Source: three-view drawing plus pictorial views. Frame: mm from the lowest corner of the part. Coordinates: 2 decimals unless noted, no trailing zeros. Order: outer loops, then holes, each group sorted by start corner. A loop starts at its lowest first (then second) coordinate and runs counter-clockwise, first axis right, second up. Notation, with made-up numbers: (26.5, 61) -> (85.5, 61) arc R25 ccw to (85.5, 93) -> close; hole circle Ø5 at (-22.5, 69.5). An arc over 180 degrees is marked (long way). Use one line per item in the form item = value. Start each with the question number.
1) Section query B-B on y = 55. Output: boundary loops of the cut face in (x, z), then the cut area to 3 significant figures.
2) Pin query (flat end, axial travel): pin 1 (2 mm diameter, centred on y = 11.2, z = 2.5, fed in from -X). Return the tip coordinate at first contact, or that it passes through.
3) Ray query, line 1 along X through (y, z) = (26.5, 2.3); line 2 along X through (y, z) = (52, 3.3); line 3 along Y through (x, z) = (41.3, 2.5). Return the intervals inside material, ascending.
4) Section query A-A on x = 36.5. Output: boundary loops of the cut face in (y, z).
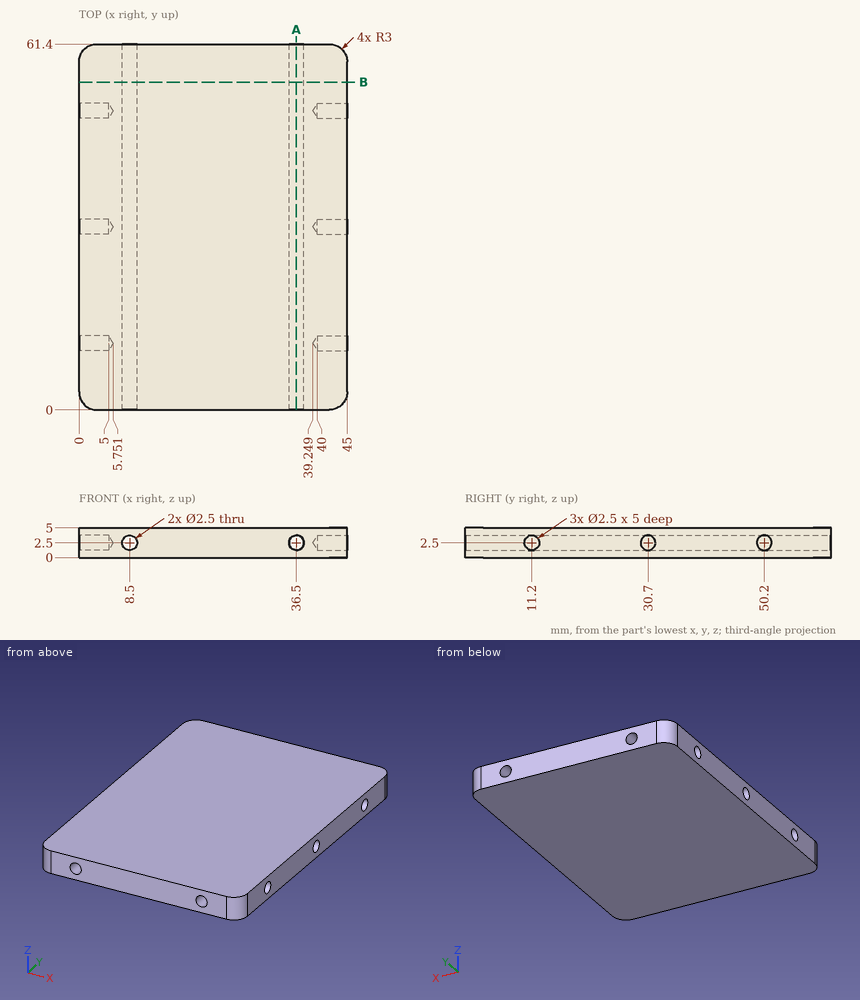
Answers below:
q1.outline = (0, 0) -> (45, 0) -> (45, 5) -> (0, 5) -> close; hole circle Ø2.5 at (8.5, 2.5); hole circle Ø2.5 at (36.5, 2.5)
q1.area = 215 mm^2
q2.pin_1 = 5.15
q3.line_1 = 0 to 7.27, 9.73 to 35.27, 37.73 to 45
q3.line_2 = 0 to 7.54, 9.46 to 35.54, 37.46 to 45
q3.line_3 = 0 to 9.95, 12.45 to 29.45, 31.95 to 48.95, 51.45 to 61.4
q4.outline = (0, 0) -> (61.4, 0) -> (61.4, 1.25) -> (0, 1.25) -> close; (0, 3.75) -> (61.4, 3.75) -> (61.4, 5) -> (0, 5) -> close
